Here's how the part is built. I have some questions about the finished solid (model axes, mm). Give positions to 0.01 mm unless a question says otherwise; leave off trailing zeros. Loops run counter-clockwise (first coordinate to the right, second up) from the corner with the lowest first, then second, coordinate; pieces in that order, holes last.
Q1. Suppose I cut it at B-B (x = -491.5). List the corners of the cut face in (y, z) for me.
Q2. I need wall thicknesses on probe 1 along X at (y, z) = (407.5, 3.5); probe 2 along Y at (x, z) = (-10, 4); probe 3 along X at (y, z) = (430, 7). Which ranges of each line are inside material? Lowest first, please.
Q3. Suppose I cut it at C-C (z = 6.5). Count the separate pieces of the cut face and the enclosed holes in it, and give its area (3 significant figures).
Q4. Suppose I cut it at A-A (y = 250). List the corners of the cut face in (x, z) for me, and give its area (3 significant figures).
Q5. I'm going to push a flat-ended pin straight in: P1, Ø6, axis at x = -630, y = 32.5, coming from the +Z side. Where does the tip first touch, or does it pass through?
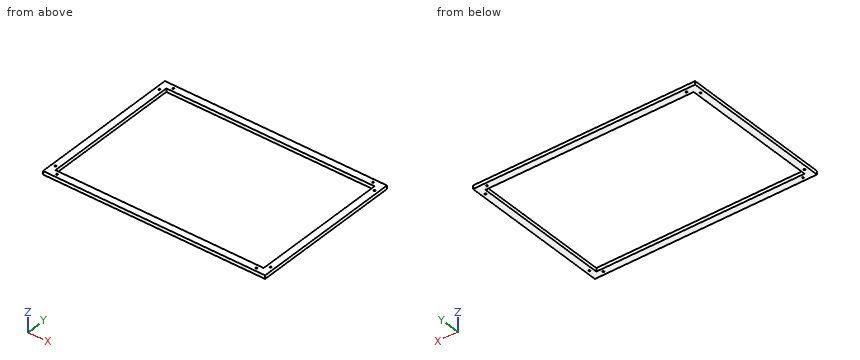
```python
from build123d import *

# Parameters (mm, degrees)
ESQUISSE1_W             = 640
ESQUISSE1_H             = 440
ESQUISSE1_W_2           = 600
ESQUISSE1_H_2           = 400
BOSS_EXTRU_1_DEPTH      = 10
ESQUISSE2_R             = 2.25
ENL_V_MAT_EXTRU_1_DEPTH = 11


with BuildPart() as part:
    # Esquisse1 → Boss.-Extru.1 (new body)
    with BuildSketch(Plane.XY):
        with Locations((-320, 220)):
            Rectangle(ESQUISSE1_W, ESQUISSE1_H)
        with Locations((-320, 220)):
            Rectangle(ESQUISSE1_W_2, ESQUISSE1_H_2, mode=Mode.SUBTRACT)
    extrude(amount=BOSS_EXTRU_1_DEPTH)

    # Esquisse2 → Enlèv. mat.-Extru.1 (cut, through all)
    with BuildSketch(Plane.XY.offset(10)):
        with Locations((-32.5, 430)):
            Circle(ESQUISSE2_R)
        with Locations((-10, 407.5)):
            Circle(ESQUISSE2_R)
        with Locations((-607.5, 430)):
            Circle(ESQUISSE2_R)
        with Locations((-630, 407.5)):
            Circle(ESQUISSE2_R)
        with Locations((-630, 32.5)):
            Circle(ESQUISSE2_R)
        with Locations((-607.5, 10)):
            Circle(ESQUISSE2_R)
        with Locations((-32.5, 10)):
            Circle(ESQUISSE2_R)
        with Locations((-10, 32.5)):
            Circle(ESQUISSE2_R)
    extrude(amount=-ENL_V_MAT_EXTRU_1_DEPTH, mode=Mode.SUBTRACT)


solid = part.part
```
Solutions:
1. outline: (0, 0) - (20, 0) - (20, 10) - (0, 10) - close; (420, 0) - (440, 0) - (440, 10) - (420, 10) - close
2. probe 1: x = -640 to -632.25, -627.75 to -620, -20 to -12.25, -7.75 to 0
2. probe 2: y = 0 to 30.25, 34.75 to 405.25, 409.75 to 440
2. probe 3: x = -640 to -609.75, -605.25 to -34.75, -30.25 to 0
3. separate pieces: 1
3. enclosed holes: 9
3. area: 41,500 mm2
4. outline: (-640, 0) - (-620, 0) - (-620, 10) - (-640, 10) - close; (-20, 0) - (0, 0) - (0, 10) - (-20, 10) - close
4. area: 400 mm2
5. P1: stops at z = 10
